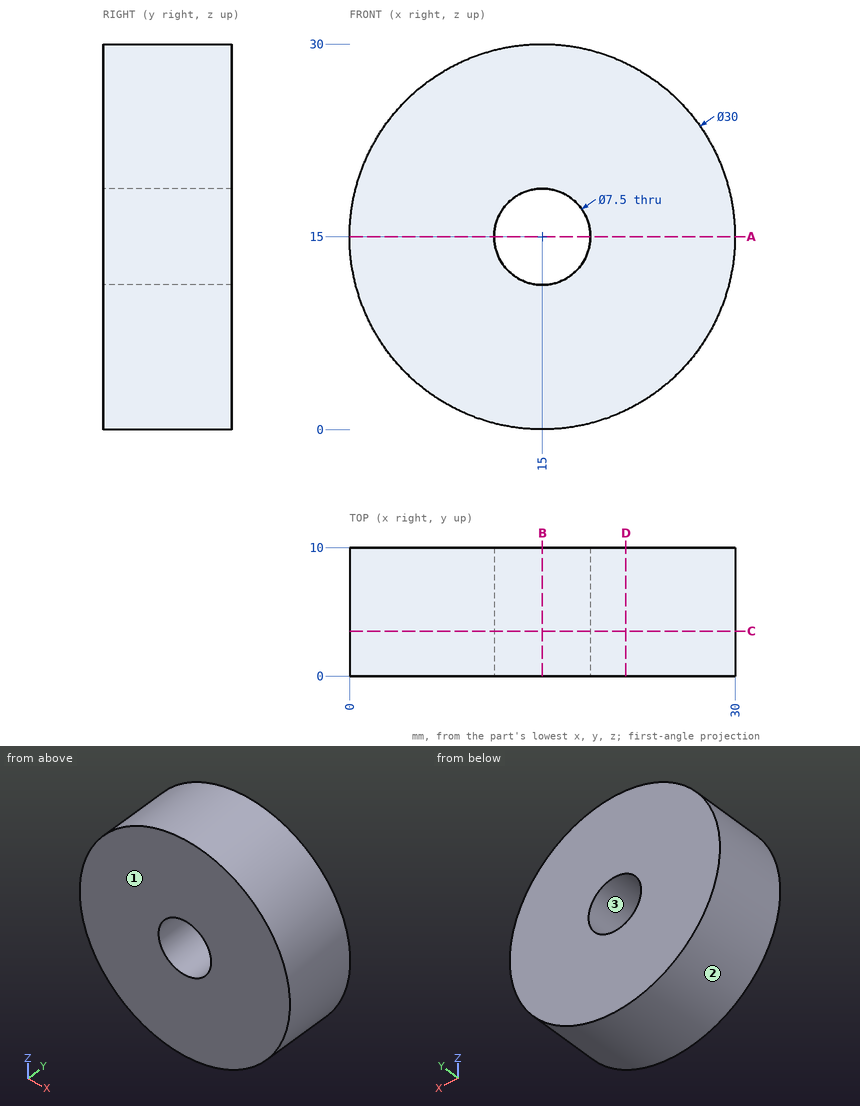
Verification items for this drawing (mm, ordinates from the low corner). Give positions to 0.01 mm unless a question says otherwise; leave off trailing zeros. Loops run counter-clockwise (first coordinate to the right, second up) from the corner with the lowest first, then second, coordinate; pieces in that order, holes last. Notation, with made-up numbers: M 52.5,5 L 102.5,5 A23 cw 102.5,35 Z; hole C 74.5,-3.75 d4. An arc over 180 degrees is marked long. Answer as a JSON object with one key per item and string values. Group by question number.
Q1. Cross-section at A-A on z = 15. Record the cut outline in (x, y), then the cut area to 3 significant figures.
Q2. Material ranges on line 1 along X through (y, z) = (6.75, 15); line 2 along X through (y, z) = (3.5, 13), recorded low to high. Write a range as [from, to].
Q3. Go/stop test with flat-tipped pins: P1, Ø6, axis at x = 15, z = 15, coming from the +Y side; P2, Ø1.5, axis at x = 26, y = 3, coming from the +Z side; P3, Ø1, axis at y = 7.5, z = 11.5, coming from the -X side; P4, Ø5, axis at x = 25, y = 1, coming from the -Z side. Record where each tip stops, or that it passes through.
Q4. Release check for a two-part mould opening along Z. For the marked faces 1, 2 and 3 record: released by +Z, released by -Z, zero draft, split by the parting line, or undercut.
Q5. Cross-section at D-D on x = 21.5. Record the cut outline in (y, z).
Q6. Cross-section at C-C on y = 3.5. Record the cut outline in (x, z).
Q7. Cross-section at B-B on x = 15. Record the cut outline in (y, z), then the cut area to 3 significant figures.
Evaluation:
{
 "1": {"outline": "M 0,0 L 11.25,0 L 11.25,10 L 0,10 Z; M 18.75,0 L 30,0 L 30,10 L 18.75,10 Z", "area": "225 mm2"},
 "2": {"line 1": "x = [0, 11.25], [18.75, 30]", "line 2": "x = [0.13, 11.83], [18.17, 29.87]"},
 "3": {"P1": "passes through", "P2": "stops at z = 25.95", "P3": "stops at x = 0.3", "P4": "stops at z = 2.01"},
 "4": {"face 1": "zero draft", "face 2": "split by the parting line", "face 3": "undercut"},
 "5": {"outline": "M 0,1.48 L 10,1.48 L 10,28.52 L 0,28.52 Z"},
 "6": {"outline": "C 15,15 d30; hole C 15,15 d7.5"},
 "7": {"outline": "M 0,0 L 10,0 L 10,11.25 L 0,11.25 Z; M 0,18.75 L 10,18.75 L 10,30 L 0,30 Z", "area": "225 mm2"}
}
